Verification items for the finished model (mm, model axes). Face numbers are marked on the shaded views. A direction names the side the tool comes from. Give positions to 0.01 mm unless a question says otherwise; leave off trailing zeros. Write each loop counter-clockwise with the first axis right and the second up, starting at its lowest first coordinate (ties: lowest second). Pieces come first, ordered by that corner, then holes. Notation, with made-up numbers: (34.25, 62.5) -> (63.25, 62.5) arc R27 ccw to (63.25, 90.5) -> close; hole circle Ø1 at (48, 79.5). An arc over 180 degrees is marked (long way). Use CSV: the item, a comma, the result in double quotes. Start each with the question number.
```python
from build123d import *

# Parameters (mm, degrees)
F0_W     = 7.874
F0_H     = 6.35
F1_DEPTH = 10.16
F2_R     = 1.905
F3_DEPTH = 10.161
F5_DEPTH = 60.325


with BuildPart() as f1:
    # F0 (on Front) → F1 (new body)
    with BuildSketch(Plane.XZ):
        Rectangle(F0_W, F0_H)
        with BuildLine():
            Line((3.937, -3.175), (-3.937, -3.175))
            ThreePointArc((-3.937, -3.175), (0, -7.112), (3.937, -3.175))
        make_face()
    extrude(amount=F1_DEPTH)

    # F2 (on face) → F3 (cut, through all)
    with BuildSketch(Plane.XZ.offset(10.16)):
        Circle(F2_R)
    extrude(amount=-F3_DEPTH, mode=Mode.SUBTRACT)

    # F4 (on face) → F5 (join)
    with BuildSketch(Plane.XY.offset(3.175)):
        with BuildLine():
            ThreePointArc((-3.937, -5.08), (0, -9.017), (3.937, -5.08))
            ThreePointArc((3.937, -5.08), (0, -1.143), (-3.937, -5.08))
        make_face()
    extrude(amount=F5_DEPTH)


solid = f1.part
```
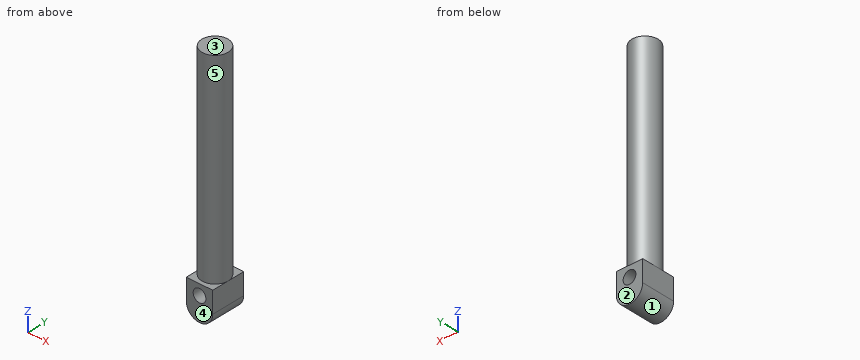
(1) Section check C-C on y = -4. Record the cut outline in (x, z) (3 decimals).
(2) Set-up check for the marked faces 4 and 5: record each of +Z, -Z, +X, -X, +Y, -Y from which the full face is reachable in a straight line by a thin tool's end or side.
(3) Draft check along Z on the marked faces 1, 2 and 3. Enter one of: released by +Z, released by -Z, zero draft, split by the parting line, or undercut.
(4) Go/stop test with flat-tipped pins: pin 1 (1.5 mm diameter, centred on x = -1, y = -3, fed in from -Z); pin 2 (2.5 mm diameter, centred on x = 0, z = 0, fed in from -Y). Record where each tip stops, or that it passes through.
(5) Section check B-B on x = 0. Record the cut outline in (y, z) (3 decimals).
(6) Section check A-A on z = 0. Record the cut outline in (x, y) (3 decimals).
(7) Section check D-D on x = 3.25. Record the cut outline in (y, z) (3 decimals).
(8) Thickness scan on line 1 (Z direction, x = 0, y = -5) (3 decimals); line 2 (Y direction, x = -0.25, z = 23.5); line 3 (Z direction, x = 1.25, y = -2.75). Record the ranges inside material, lowest first. Write a range as from..to.
Data:
1,outline,"(-3.937, -3.175) arc R3.937 ccw to (3.937, -3.175) -> (3.937, 3.175) -> (3.786, 3.175) -> (3.786, 63.5) -> (-3.786, 63.5) -> (-3.786, 3.175) -> (-3.937, 3.175) -> close; hole circle Ø3.81 at (0, 0)"
2,face 4,"+Z, -Z, +X, -X, -Y"
2,face 5,"+Z"
3,face 1,"released by -Z"
3,face 2,"zero draft"
3,face 3,"released by +Z"
4,pin 1,"stops at z = -7.1"
4,pin 2,"passes through"
5,outline,"(-10.16, -7.112) -> (0, -7.112) -> (0, -1.905) -> (-10.16, -1.905) -> close; (-10.16, 1.905) -> (0, 1.905) -> (0, 3.175) -> (-1.143, 3.175) -> (-1.143, 63.5) -> (-9.017, 63.5) -> (-9.017, 3.175) -> (-10.16, 3.175) -> close"
6,outline,"(-3.937, -10.16) -> (-1.905, -10.16) -> (-1.905, 0) -> (-3.937, 0) -> close; (1.905, -10.16) -> (3.937, -10.16) -> (3.937, 0) -> (1.905, 0) -> close"
7,outline,"(-10.16, -5.397) -> (0, -5.397) -> (0, 3.175) -> (-2.858, 3.175) -> (-2.858, 63.5) -> (-7.302, 63.5) -> (-7.302, 3.175) -> (-10.16, 3.175) -> close"
8,line 1,"z = -7.112..-1.905, 1.905..63.5"
8,line 2,"y = -9.01..-1.15"
8,line 3,"z = -6.91..-1.44, 1.44..63.5"
